Can you work these out from the model? Positions are in its coordinate system, mm. A direction names the side the tool comes from. Coordinates: 2 decimals unless noted, no trailing zeros. Order: outer loops, then holes, each group sorted by start corner. A loop starts at its lowest first (then second) coordinate and runs counter-clockwise, first axis right, second up. Notation, with made-up numbers: (38.25, 68) -> (94.25, 68) arc R19 ccw to (94.25, 77) -> close; hole circle Ø7 at (-31, 88.5). An arc over 180 degrees is marked (long way). Answer as CSV lines item,"result".
from build123d import *

# Parameters (mm, degrees)
SKETCH1_R           = 8
BOSS_EXTRUDE1_DEPTH = 95
SKETCH2_R           = 4
CUT_EXTRUDE1_DEPTH  = 45
SKETCH4_W           = 2.279315198
SKETCH4_H           = 4.278597429
SKETCH4_H_2         = 4.06286311
CUT_EXTRUDE2_DEPTH  = 40
BOSS_EXTRUDE2_DEPTH = 15
SKETCH6_R           = 5
BOSS_EXTRUDE3_DEPTH = 15


with BuildPart() as part:
    # Sketch1 → Boss-Extrude1 (new body)
    with BuildSketch(Plane(origin=(0, 0, 0), x_dir=(1, 0, 0), z_dir=(0, 1, 0))):
        with Locations(Location((0, 0, 0), (0, 0, 270))):
            Circle(SKETCH1_R)
    extrude(amount=BOSS_EXTRUDE1_DEPTH)

    # Sketch2 → Cut-Extrude1 (cut)
    with BuildSketch(Plane.XZ):
        with Locations(Location((0, 0, 0), (0, 0, 270))):
            Circle(SKETCH2_R)
    extrude(amount=-CUT_EXTRUDE1_DEPTH, mode=Mode.SUBTRACT)

    # Sketch4 → Cut-Extrude2 (cut)
    with BuildSketch(Plane(origin=(0, 95, 0), x_dir=(1, 0, 0), z_dir=(0, 1, 0))):
        with BuildLine():
            Line((1.275256108, 4.278597429), (-0.547648504, 4.278597429))
            Line((-0.547648504, 4.278597429), (-0.547648504, 0))
            Line((-0.547648504, 0), (1.67579289, 0))
            ThreePointArc((1.67579289, 0), (3.423908341, 2.321694794), (1.275256108, 4.278597429))
        make_face()
        with Locations((-1.687306103, 2.139298715)):
            Rectangle(SKETCH4_W, SKETCH4_H)
        with Locations((-1.687306103, -2.031431555)):
            Rectangle(SKETCH4_W, SKETCH4_H_2)
        Polygon((1.67579289, 0), (-0.547648504, 0), (1.653720681, -4.06286311), (3.877162075, -4.06286311), align=None)
    extrude(amount=-CUT_EXTRUDE2_DEPTH, mode=Mode.SUBTRACT)

    # Sketch5 → Boss-Extrude2 (add)
    with BuildSketch(Plane(origin=(0, 0, 0), x_dir=(1, 0, 0), z_dir=(0, 1, 0))):
        with BuildLine():
            ThreePointArc((-62.501736138, 39.996744571), (-65.482019756, 31.895818698), (-73.001736138, 27.657781892))
            Line((-73.001736138, 27.657781892), (-73.001736138, 27.496744571))
            Line((-73.001736138, 27.496744571), (-3.57279106, -7.157874268))
            ThreePointArc((-3.57279106, -7.157874268), (-7.025809748, 3.825963588), (4.074261757, 6.884794197))
            Line((4.074261757, 6.884794197), (-65.396568509, 47.996166726))
            ThreePointArc((-65.396568509, 47.996166726), (-63.247702886, 44.250296301), (-62.501736138, 39.996744571))
        make_face()
        with BuildLine():
            ThreePointArc((-72.612195867, 52.266222852), (-72.806691043, 52.302506515), (-73.001736138, 52.33570725))
            Line((-73.001736138, 52.33570725), (-73.001736138, 27.657781892))
            ThreePointArc((-73.001736138, 27.657781892), (-65.482019756, 31.895818698), (-62.501736138, 39.996744571))
            ThreePointArc((-62.501736138, 39.996744571), (-63.247702886, 44.250296301), (-65.396568509, 47.996166726))
            Line((-65.396568509, 47.996166726), (-72.612195867, 52.266222852))
        make_face()
    extrude(amount=BOSS_EXTRUDE2_DEPTH)

    # Sketch6 → Boss-Extrude3 (add)
    with BuildSketch(Plane(origin=(0, 15, 0), x_dir=(1, 0, 0), z_dir=(0, 1, 0))):
        with Locations(Location((-48.001736138, 26.246610631, 0), (0, 0, 270))):
            Circle(SKETCH6_R)
    extrude(amount=BOSS_EXTRUDE3_DEPTH)

    # Sketch8 → Cut-Revolve1 (revolve, cut)
    with BuildSketch(Plane(origin=(0, 0, 0), x_dir=(-0.4149509310359906, 0, 0.909843791445743), z_dir=(0.909843791445743, 0, 0.4149509310359906)), mode=Mode.PRIVATE) as cut_revolve1_sk:
        Polygon((0, -45), (-4.166361625, -45), (0, -52.216350017), align=None)
    revolve(cut_revolve1_sk.sketch.rotate(Axis((0, 52.216350017, 0), (0, -1, 0)), 6.099837448), axis=Axis((0, 52.216350017, 0), (0, -1, 0)), mode=Mode.SUBTRACT)


solid = part.part
Q1. Imagine slicing it at C-C (y = 18). List the corners of the cut face in (x, z) for me.
Solution:
outline,"circle Ø10 at (-48, -26.25); circle Ø16 at (0, 0); hole circle Ø8 at (0, 0)"
Q2. Imagine slicing it at A-A (y = 7). List the corners of the cut face in (x, z) for me.
Solution:
outline,"(-73, -52.34) arc R12.5 ccw to (-72.61, -52.27) -> (4.07, -6.88) arc R8 ccw to (-3.57, 7.16) -> (-73, -27.5) -> close; hole circle Ø8 at (0, 0)"
Q3. Imagine slicing it at B-B (z = -29.5). List the corners of the cut face in (x, y) for me, and give its area (3 significant figures).
Solution:
outline,"(-73, 0) -> (-34.14, 0) -> (-34.14, 15) -> (-44.2, 15) -> (-44.2, 30) -> (-51.8, 30) -> (-51.8, 15) -> (-73, 15) -> close"
area,"697 mm2"
Q4. If I drill on line 1 (X direction, y = 30, z = 0); line 2 (Y direction, x = -49, z = -19); line 3 (X direction, y = 14, z = 0), over which ranges is the centre line in solid material (lowest first)?
Solution:
line 1,"-8 to -4, 4 to 8"
line 2,"0 to 15"
line 3,"-17.91 to -4, 4 to 8"
Q5. Imagine slicing it at D-D (x = -50). List the corners of the cut face in (y, z) for me.
Solution:
outline,"(0, -38.88) -> (15, -38.88) -> (15, -30.83) -> (30, -30.83) -> (30, -21.66) -> (15, -21.66) -> (15, -16.02) -> (0, -16.02) -> close"
Q6. Which directions (+Z, -Z, +X, -X, +Y, -Y) give clear straight access to the entire face, cutting with the end or side of a thin tool? Please do faces 1 (the cylindrical face through (-3.905, 22.185, 0.867)), 2 (the flat face through (-48, 30, -26)), 3 (the flat face through (-2, 75, 4.063)).
Solution:
face 1,"-Y"
face 2,"+Z, -Z, +X, -X, +Y"
face 3,"+Y"
Q7. We'd pull the mould along Z, two halves only. Please class faces 4 (the cylindrical face through (6.746, 46.835, 4.301)), 5 (the flat face through (-73.002, 7, -40)), 6 (the conical face through (0.224, 49.461, -1.575)): pulls with the +Z half, pulls with the -Z half, needs draft (parallel to the pull), parting line crosses it, or undercut.
Solution:
face 4,"parting line crosses it"
face 5,"needs draft"
face 6,"undercut"
Q8. For P1, Ø12, axis at y = 32.5, z = -39.5, coming from the +X side; P2, Ø1.1, axis at x = 3, y = 74, coming from the -Z side; P3, Ø3.5, axis at y = 68, z = 2.5, coming from the -X side; P4, Ø8, axis at x = -52.5, z = -16.5, coming from the +Y side, each with a flat end and sliding along its axis, tell me the tip position at first contact or that it passes through.
Solution:
P1,"through"
P2,"z = -7.62"
P3,"x = -7.96"
P4,"y = 15"
